Read the model definition and answer for the solid it produces. Units are mm, in the model's axes. Coordinates: 2 decimals unless noted, no trailing zeros. Write each loop counter-clockwise with the first axis right and the second up, starting at its lowest first coordinate (ties: lowest second). Pieces come first, ordered by that corner, then holes. Notation, with made-up numbers: (-37, 41.5) -> (-20, 41.5) arc R25 ccw to (-20, 79.5) -> close; hole circle Ø1 at (13, 63). An arc over 180 degrees is marked (long way). One line per item, written item: value. Start each with the question number.
1. Find section C-C, the plane x = -412.5. Write down the section's boundary in (y, z) (3 decimals).
2. Find section A-A, the plane z = 303. Write down the section's boundary in (x, y), and give its area (3 significant figures).
3. Find section B-B, the plane y = -20. Write down the section's boundary in (x, z) (3 decimals), and give its area (3 significant figures).
4. Consider line 1 along Z through (x, y) = (549, -12) (3 decimals); line 2 along X through (y, z) = (-25, 273.5). Determine where each line is inside the solid, lowest interval first.
```python
from build123d import *

# Parameters (mm, degrees)
F0_W     = 2387.6
F0_H     = 31.75
F1_DEPTH = 31.75
F2_W     = 31.75
F2_H     = 31.75
F3_DEPTH = 469.9
F4_W     = 31.75
F4_H     = 31.75
F5_DEPTH = 2355.85
F6_W     = 31.75
F6_H     = 31.75
F7_DEPTH = 501.65
F8_W     = 31.75
F8_H     = 31.75
F9_DEPTH = 2336.8


with BuildPart() as f1:
    # F0 (on Front) → F1 (new body)
    with BuildSketch(Plane.XZ):
        Rectangle(F0_W, F0_H)
    extrude(amount=F1_DEPTH)

    # F2 (on face) → F3 (join)
    with BuildSketch(Plane.XY.offset(15.875)):
        with Locations((-1177.925, -15.875)):
            Rectangle(F2_W, F2_H)
    extrude(amount=F3_DEPTH)

    # F4 (on face) → F5 (join)
    with BuildSketch(Plane.YZ.offset(-1162.05)):
        with Locations((-15.875, 469.9)):
            Rectangle(F4_W, F4_H)
    extrude(amount=F5_DEPTH)

    # F6 (on face) → F7 (join)
    with BuildSketch(Plane.XY.offset(485.775)):
        with Locations((1177.925, -15.875)):
            Rectangle(F6_W, F6_H)
    extrude(amount=-F7_DEPTH)

    # F8 (on face) → F9 (join)
    with BuildSketch(Plane.YZ.offset(-1162.05)):
        with Locations((-15.875, 164.438751)):
            Rectangle(F8_W, F8_H)
    extrude(amount=F9_DEPTH)


solid = f1.part
```
Answer block:
1. outline: (-31.75, -15.875) -> (0, -15.875) -> (0, 15.875) -> (-31.75, 15.875) -> close; (-31.75, 148.564) -> (0, 148.564) -> (0, 180.314) -> (-31.75, 180.314) -> close; (-31.75, 454.025) -> (0, 454.025) -> (0, 485.775) -> (-31.75, 485.775) -> close
2. outline: (-1193.8, -31.75) -> (-1162.05, -31.75) -> (-1162.05, 0) -> (-1193.8, 0) -> close; (1162.05, -31.75) -> (1193.8, -31.75) -> (1193.8, 0) -> (1162.05, 0) -> close
2. area: 2,020 mm2
3. outline: (-1193.8, -15.875) -> (1193.8, -15.875) -> (1193.8, 485.775) -> (-1193.8, 485.775) -> close; hole (-1162.05, 15.875) -> (1162.05, 15.875) -> (1162.05, 148.564) -> (-1162.05, 148.564) -> close; hole (-1162.05, 180.314) -> (1162.05, 180.314) -> (1162.05, 454.025) -> (-1162.05, 454.025) -> close
3. area: 253,000 mm2
4. line 1: z = -15.875 to 15.875, 148.564 to 180.314, 454.025 to 485.775
4. line 2: x = -1193.8 to -1162.05, 1162.05 to 1193.8
